```python
from build123d import *

# Parameters (mm, degrees)
SKETCH1_W           = 50.8
SKETCH1_H           = 76.2
BOSS_EXTRUDE1_DEPTH = 50.8
SKETCH2_R           = 19.812
CUT_EXTRUDE1_DEPTH  = 51.8
SKETCH3_R           = 6.35
CUT_EXTRUDE2_DEPTH  = 51.8


with BuildPart() as part:
    # Sketch1 → Boss-Extrude1 (new body)
    with BuildSketch(Plane.XY):
        Rectangle(SKETCH1_W, SKETCH1_H)
    extrude(amount=BOSS_EXTRUDE1_DEPTH)

    # Sketch2 → Cut-Extrude1 (cut, through all)
    with BuildSketch(Plane.XY.offset(50.8)):
        with Locations((0, 16.51)):
            Circle(SKETCH2_R)
    extrude(amount=-CUT_EXTRUDE1_DEPTH, mode=Mode.SUBTRACT)

    # Sketch3 → Cut-Extrude2 (cut, through all)
    with BuildSketch(Plane(origin=(25.4, 0, 0), x_dir=(0, 0, -1), z_dir=(1, 0, 0))):
        with Locations((-25.4, -25.4)):
            Circle(SKETCH3_R)
    extrude(amount=-CUT_EXTRUDE2_DEPTH, mode=Mode.SUBTRACT)


solid = part.part
```
Work out the finished part from the listing and answer in its coordinate system (mm). Round coordinates to 2 decimals unless told otherwise and drop trailing zeros. Order: outer loops, then holes, each group sorted by start corner. A loop starts at its lowest first (then second) coordinate and runs counter-clockwise, first axis right, second up.
Q1. The mould has two halves that part along Z. Classify faces 1 (the flat face through (-25.4, -1, 25)), 2 (the flat face through (0, -8, 0)), 3 (the cylindrical face through (0.356, -31.034, 22.47)), 4 (the flat face through (0, -8, 50.8)): pulls with the +Z half, pulls with the -Z half, needs draft (parallel to the pull), parting line crosses it, or undercut.
Solution:
face 1: needs draft
face 2: pulls with the -Z half
face 3: undercut
face 4: pulls with the +Z half
Q2. A cutting plane is placed at B-B, the plane x = 3.5. Determine the outline of the cut face in (y, z).
Solution:
outline: (-38.1, 0) - (-2.99, 0) - (-2.99, 50.8) - (-38.1, 50.8) - close; (36.01, 0) - (38.1, 0) - (38.1, 50.8) - (36.01, 50.8) - close; hole circle Ø12.7 at (-25.4, 25.4)
Q3. Given pin 1 Ø10 at (y, z) = (-25.4, 25.4) entering from +X, flat-ended and moving along its own axis, determine where the tip first touches the part or whether it passes through.
Solution:
pin 1: passes through
Q4. A cutting plane is placed at D-D, the plane z = 13. Determine the outline of the cut face in (x, y).
Solution:
outline: (-25.4, -38.1) - (25.4, -38.1) - (25.4, 38.1) - (-25.4, 38.1) - close; hole circle Ø39.62 at (0, 16.51)
Q5. A cutting plane is placed at A-A, the plane z = 25.4. Determine the outline of the cut face in (x, y).
Solution:
outline: (-25.4, -38.1) - (25.4, -38.1) - (25.4, -31.75) - (-25.4, -31.75) - close; (-25.4, -19.05) - (25.4, -19.05) - (25.4, 38.1) - (-25.4, 38.1) - close; hole circle Ø39.62 at (0, 16.51)
Q6. Find the intervals of material crossed by line 1 along Z through (x, y) = (2, -25); line 2 along X through (y, z) = (16.5, 13.5); line 3 along Y through (x, z) = (0, 26), in increasing order.
Solution:
line 1: z = 0 to 19.06, 31.74 to 50.8
line 2: x = -25.4 to -19.81, 19.81 to 25.4
line 3: y = -38.1 to -31.72, -19.08 to -3.3, 36.32 to 38.1
Q7. A cutting plane is placed at C-C, the plane y = -25.4. Determine the outline of the cut face in (x, z).
Solution:
outline: (-25.4, 0) - (25.4, 0) - (25.4, 19.05) - (-25.4, 19.05) - close; (-25.4, 31.75) - (25.4, 31.75) - (25.4, 50.8) - (-25.4, 50.8) - close
